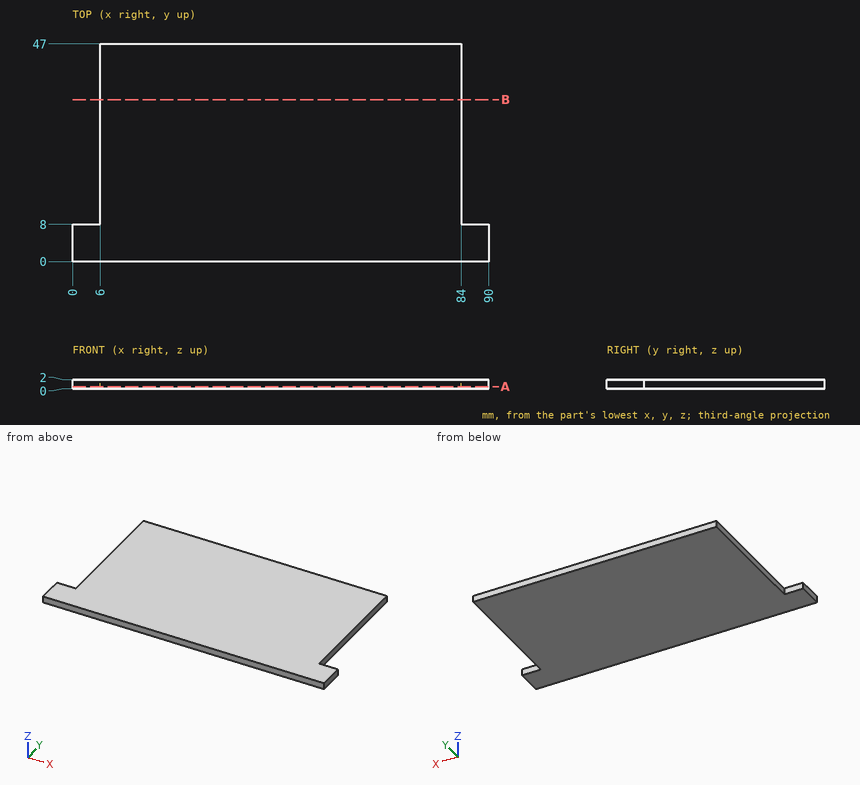
Geometry: see drawing. Coordinates: mm, zero at the bounding-box minimum. Round coordinates to 2 decimals unless told otherwise and drop trailing zeros. Write each loop counter-clockwise with the first axis right and the second up, starting at its lowest first coordinate (ties: lowest second). Pieces come first, ordered by that corner, then holes. Notation, with made-up numbers: M 16.25,-13 L 20.25,-13 A20 cw 20.25,23 Z; hole C 44.5,23.25 d4. An arc over 180 degrees is marked long. Answer as a JSON object with one key per item and string values. Group by question number.
(1) Section query A-A on z = 0.45. Output: boundary loops of the cut face in (x, y), then the cut area to 3 significant figures.
(2) Ray query, line 1 (X direction, y = 11, z = 1.65). Return the intervals inside material, ascending. Write a range as [from, to].
(3) Section query B-B on y = 35. Output: boundary loops of the cut face in (x, z), then the cut area to 3 significant figures.
(4) First-contact query: pin 1 (1 mm diameter, centred on x = 88, z = 1, fed in from +Y); pin 2 (1 mm diameter, centred on y = 26, z = 1.5, fed in from +X). Flat tips, straight axial feed; report the tip coordinate or a pass-through.
Computed values:
{
 "1": {"outline": "M 0,0 L 90,0 L 90,8 L 84,8 L 84,47 L 6,47 L 6,8 L 0,8 Z", "area": "3,760 mm^2"},
 "2": {"line 1": "[6, 84]"},
 "3": {"outline": "M 6,0 L 84,0 L 84,2 L 6,2 Z", "area": "156 mm^2"},
 "4": {"pin 1": "y = 8", "pin 2": "x = 84"}
}
